```python
from build123d import *

# Parameters (mm, degrees)
SKETCH1_W           = 120
SKETCH1_H           = 84
SKETCH1_W_2         = 115.6
SKETCH1_H_2         = 80
BOSS_EXTRUDE1_DEPTH = 155
FILLET1_R           = 4
SKETCH3_W           = 2
SKETCH3_H           = 2.5
SKETCH3_W_2         = 2.5
SKETCH3_H_2         = 2
FINALBOX_DEPTH      = 155


with BuildPart() as part:
    # Sketch1 → Boss-Extrude1 (new body)
    with BuildSketch(Plane.XY):
        Rectangle(SKETCH1_W, SKETCH1_H)
        Rectangle(SKETCH1_W_2, SKETCH1_H_2, mode=Mode.SUBTRACT)
    extrude(amount=BOSS_EXTRUDE1_DEPTH)

    # Fillet1
    fillet1_edges = [part.edges().sort_by_distance(p)[0] for p in [
        (60, -42, 77.5),
        (-60, -42, 77.5),
        (-60, 42, 77.5),
        (60, 42, 77.5),
    ]]
    fillet(fillet1_edges, radius=FILLET1_R)

    # Sketch3 → FinalBox (add, through all)
    with BuildSketch(Plane.XY.offset(155)):
        with Locations((-53.8, 38.75)):
            Rectangle(SKETCH3_W, SKETCH3_H)
        with Locations((-49.8, 38.75)):
            Rectangle(SKETCH3_W, SKETCH3_H)
        with Locations((-45.8, 38.75)):
            Rectangle(SKETCH3_W, SKETCH3_H)
        with Locations((-56.55, 35.4)):
            Rectangle(SKETCH3_W_2, SKETCH3_H_2)
        with Locations((-56.55, 31.4)):
            Rectangle(SKETCH3_W_2, SKETCH3_H_2)
        with Locations((-56.55, 27.4)):
            Rectangle(SKETCH3_W_2, SKETCH3_H_2)
        with Locations((56.55, 27.4)):
            Rectangle(SKETCH3_W_2, SKETCH3_H_2)
        with Locations((56.55, 31.4)):
            Rectangle(SKETCH3_W_2, SKETCH3_H_2)
        with Locations((56.55, 35.4)):
            Rectangle(SKETCH3_W_2, SKETCH3_H_2)
        with Locations((53.8, 38.75)):
            Rectangle(SKETCH3_W, SKETCH3_H)
        with Locations((49.8, 38.75)):
            Rectangle(SKETCH3_W, SKETCH3_H)
        with Locations((45.8, 38.75)):
            Rectangle(SKETCH3_W, SKETCH3_H)
        with Locations((45.8, -38.75)):
            Rectangle(SKETCH3_W, SKETCH3_H)
        with Locations((49.8, -38.75)):
            Rectangle(SKETCH3_W, SKETCH3_H)
        with Locations((53.8, -38.75)):
            Rectangle(SKETCH3_W, SKETCH3_H)
        with Locations((56.55, -35.4)):
            Rectangle(SKETCH3_W_2, SKETCH3_H_2)
        with Locations((56.55, -31.4)):
            Rectangle(SKETCH3_W_2, SKETCH3_H_2)
        with Locations((56.55, -27.4)):
            Rectangle(SKETCH3_W_2, SKETCH3_H_2)
        with Locations((-45.8, -38.75)):
            Rectangle(SKETCH3_W, SKETCH3_H)
        with Locations((-49.8, -38.75)):
            Rectangle(SKETCH3_W, SKETCH3_H)
        with Locations((-53.8, -38.75)):
            Rectangle(SKETCH3_W, SKETCH3_H)
        with Locations((-56.55, -35.4)):
            Rectangle(SKETCH3_W_2, SKETCH3_H_2)
        with Locations((-56.55, -31.4)):
            Rectangle(SKETCH3_W_2, SKETCH3_H_2)
        with Locations((-56.55, -27.4)):
            Rectangle(SKETCH3_W_2, SKETCH3_H_2)
        with Locations((-4, -38.75)):
            Rectangle(SKETCH3_W, SKETCH3_H)
        with Locations((-4, 38.75)):
            Rectangle(SKETCH3_W, SKETCH3_H)
        with Locations((0, 38.75)):
            Rectangle(SKETCH3_W, SKETCH3_H)
        with Locations((4, 38.75)):
            Rectangle(SKETCH3_W, SKETCH3_H)
        with Locations((0, -38.75)):
            Rectangle(SKETCH3_W, SKETCH3_H)
        with Locations((4, -38.75)):
            Rectangle(SKETCH3_W, SKETCH3_H)
    extrude(amount=-FINALBOX_DEPTH)


solid = part.part
```
Read the model definition and answer for the solid it produces. Units are mm, in the model's axes. A direction names the side the tool comes from. Give positions to 0.01 mm unless a question says otherwise; leave off trailing zeros. Order: outer loops, then holes, each group sorted by start corner. A loop starts at its lowest first (then second) coordinate and runs counter-clockwise, first axis right, second up.
(1) Given pin 1 (1.2 mm diameter, centred on x = -57, z = 41, fed in from -Y); pin 2 (0.8 mm diameter, centred on y = -39, z = 72, fed in from +X), each flat-ended and moving along its own axis, determine where each tip first touches the part or whether it passes through.
(2) Find section A-A (y = -9). Give the vertices of the cut face in (x, z), plus the area to 3 significant figures.
(3) For faces 1 (the flat face through (25, -40, 76)), 2 (the cylindrical face through (-58.859, 40.797, 78.585)), determine the directions among +Z, -Z, +X, -X, +Y, -Y from which every point of the face is accessible in a straight line to the end or side of a thin tool.
(4) Find section B-B (x = 36). Give the vertices of the cut face in (y, z).
(5) Straight lines are drawn through the part: L1, parallel to Y at x = 33, z = 21; L2, parallel to X at y = 2, z = 58; L3, parallel to Y at x = 45.5, z = 113. For each, find the intervals that lie inside material, in ascending order.
(6) For a pull along X with two mould halves and no side action, classify faces 3 (the flat face through (-57.8, -38, 76)), 4 (the cylindrical face through (-58.859, -40.797, 78.585)), 5 (the flat face through (-1, 42, 76)) as released by +X, released by -X, zero draft, split by the parting line, or undercut.
Result sheet:
1. pin 1: stops at y = -41.98
1. pin 2: stops at x = 59.95
2. outline: (-60, 0) - (-57.8, 0) - (-57.8, 155) - (-60, 155) - close; (57.8, 0) - (60, 0) - (60, 155) - (57.8, 155) - close
2. area: 682 mm2
3. face 1: +Z, -Z
3. face 2: +Z, -Z, -X, +Y
4. outline: (-42, 0) - (-40, 0) - (-40, 155) - (-42, 155) - close; (40, 0) - (42, 0) - (42, 155) - (40, 155) - close
5. L1: y = -42 to -40, 40 to 42
5. L2: x = -60 to -57.8, 57.8 to 60
5. L3: y = -42 to -37.5, 37.5 to 42
6. face 3: undercut
6. face 4: released by -X
6. face 5: zero draft
